The listing builds one solid part. Answer for the finished solid, in the listing's coordinates (mm). Give positions to 0.01 mm unless a question says otherwise; leave off trailing zeros. Loops run counter-clockwise (first coordinate to the right, second up) from the corner with the lowest first, then second, coordinate; pieces in that order, holes last. Notation, with made-up numbers: (79.5, -3) - (94.5, -3) arc R23 ccw to (94.5, 7) - close; hole circle Ø7 at (82.25, 72.5). An arc over 180 degrees is marked (long way). Write item = value, one per line. Start each with the question number.
1) The part is cut by section A-A on x = 161.5. Write down the section's boundary in (y, z), plus the area to 3 significant figures.
2) Consider probe 1 along Z at (x, y) = (45, -15.5); probe 2 along Z at (x, y) = (-182, -16.75). Determine where each line is inside the solid, lowest interval first.
3) Flat-ended cylindrical pins translate along their axes: P1, Ø1, axis at x = 155, y = -4, coming from the +Z side; P2, Ø2, axis at x = 2, y = -12.5, coming from the +Z side; P3, Ø1.5, axis at x = 133, y = -14, coming from the +Z side. Find the tip coordinate at first contact, or state that the pin passes through.
from build123d import *

# Parameters (mm, degrees)
F0_W     = 430
F0_H     = 285
F1_DEPTH = 18
F3_DEPTH = 438
F4_R     = 1
F5_R     = 1


with BuildPart() as f1:
    # F0 (on Front) → F1 (new body)
    with BuildSketch(Plane.XZ):
        Rectangle(F0_W, F0_H)
    extrude(amount=F1_DEPTH)

    # F2 (on face) → F3 (cut)
    with BuildSketch(Plane.YZ.offset(215)):
        Polygon((0, 142.5), (-18, 142.5), (0, 124.5), align=None)
    extrude(amount=-F3_DEPTH, mode=Mode.SUBTRACT)

    # F4
    f4_edges = [f1.edges().sort_by_distance(p)[0] for p in [
        (0, -18, 142.5),
    ]]
    fillet(f4_edges, radius=F4_R)

    # F5
    f5_edges = [f1.edges().sort_by_distance(p)[0] for p in [
        (-215, -18, -1.207107),
        (0, -18, -142.5),
        (215, -18, -1.207107),
    ]]
    fillet(f5_edges, radius=F5_R)


solid = f1.part
Answer below:
q1.outline = (-18, -141.5) arc R1 ccw to (-17, -142.5) - (0, -142.5) - (0, 124.5) - (-16.29, 140.79) arc R1 ccw to (-18, 140.09) - close
q1.area = 4,970 mm2
q2.probe_1 = -142.5 to 140
q2.probe_2 = -142.5 to 141.05
q3.P1 = 129
q3.P2 = 138
q3.P3 = 139.25
